Here's how the part is built. I have some questions about the finished solid (model axes, mm). A direction names the side the tool comes from. Give positions to 0.01 mm unless a question says otherwise; leave off trailing zeros. Write each loop counter-clockwise with the first axis right and the second up, starting at its lowest first coordinate (ties: lowest second). Pieces come first, ordered by that corner, then holes. Notation, with made-up numbers: (74, 76.5) -> (79, 76.5) arc R5 cw to (79, 82.5) -> close; hole circle Ø3 at (15, -17). An arc over 180 degrees is marked (long way). Use one line per item in the form item = value.
```python
from build123d import *

# Parameters (mm, degrees)
EXTRUDE_THIN1_DEPTH = 60
SKETCH2_R           = 5
CUT_EXTRUDE1_DEPTH  = 123.065556157
SKETCH3_R           = 5
CUT_EXTRUDE2_DEPTH  = 123.065556157


with BuildPart() as part:
    # Sketch1 → Extrude-Thin1 (new body)
    with BuildSketch(Plane.XY):
        Polygon((80, 0), (0, 0), (0, 70), (-6, 70), (-6, -6), (80, -6), align=None)
    extrude(amount=EXTRUDE_THIN1_DEPTH)

    # Sketch2 → Cut-Extrude1 (cut, through all)
    with BuildSketch(Plane(origin=(0, 0, 0), x_dir=(1, 0, 0), z_dir=(0, 1, 0))):
        with Locations(Location((70, -6.887679605, 0), (0, 0, 270))):
            Circle(SKETCH2_R)
        with Locations(Location((70, -51.887679605, 0), (0, 0, 270))):
            Circle(SKETCH2_R)
    extrude(amount=-CUT_EXTRUDE1_DEPTH, mode=Mode.SUBTRACT)

    # Sketch3 → Cut-Extrude2 (cut, through all)
    with BuildSketch(Plane(origin=(0, 0, 0), x_dir=(0, 0, -1), z_dir=(1, 0, 0))):
        with Locations((-30, 35)):
            Circle(SKETCH3_R)
    extrude(amount=-CUT_EXTRUDE2_DEPTH, mode=Mode.SUBTRACT)


solid = part.part
```
Q1. I want a section at A-A, the plane x = 70. Write out the boundary of the cut face in (y, z), and give its area (3 significant figures).
Result set:
outline = (-6, 0) -> (0, 0) -> (0, 1.89) -> (-6, 1.89) -> close; (-6, 11.89) -> (0, 11.89) -> (0, 46.89) -> (-6, 46.89) -> close; (-6, 56.89) -> (0, 56.89) -> (0, 60) -> (-6, 60) -> close
area = 240 mm2
Q2. If we mould it in two halves opening along Z, with no side actions, what happens to faces 1 (the face through (36, -6, 30)), 2 (the face through (18, -2, 0)), 3 (the face through (-3, 38, 34)), 4 (the face through (65.12, -2.96, 5.8))? For each: +Z half, -Z half, draft (parallel to the pull), parting line (faces both ways), or undercut.
Result set:
face_1 = draft
face_2 = -Z half
face_3 = undercut
face_4 = undercut
Q3. If I drill on line 1 along X through (y, z) = (50, 54.5); line 2 along Y through (x, z) = (-4, 30), over which ranges is the centre line in solid material (lowest first)? Write a range as from..to.
Result set:
line_1 = -6..0
line_2 = -6..30, 40..70
Q4. I want a section at B-B, the plane y = 35. Write out the boundary of the cut face in (x, z).
Result set:
outline = (-6, 0) -> (0, 0) -> (0, 25) -> (-6, 25) -> close; (-6, 35) -> (0, 35) -> (0, 60) -> (-6, 60) -> close
Q5. I want a section at C-C, the plane z = 30. Write out the boundary of the cut face in (x, y).
Result set:
outline = (-6, -6) -> (80, -6) -> (80, 0) -> (0, 0) -> (0, 30) -> (-6, 30) -> close; (-6, 40) -> (0, 40) -> (0, 70) -> (-6, 70) -> close
Q6. Which directions (+Z, -Z, +X, -X, +Y, -Y) give clear straight access to the entire face, cutting with the end or side of a thin tool? Please do faces 5 (the face through (-6, 33, 23)), 6 (the face through (41, 0, 30)).
Result set:
face_5 = +Z, -Z, -X, +Y, -Y
face_6 = +Z, -Z, +X, +Y
Q7. I want a section at D-D, the plane z = 22.5. Write out the boundary of the cut face in (x, y), and give its area (3 significant figures).
Result set:
outline = (-6, -6) -> (80, -6) -> (80, 0) -> (0, 0) -> (0, 70) -> (-6, 70) -> close
area = 936 mm2
Q8. Will these pins go through, and if not, where does the flat tip stop? pin 1 Ø2 at (y, z) = (11, 33) entering from +X; pin 2 Ø8 at (x, z) = (70, 51.89) entering from +Y; pin 3 Ø11.5 at (x, z) = (70, 6.89) entering from +Y.
Result set:
pin_1 = 0
pin_2 = through
pin_3 = 0
